```python
from build123d import *

# Parameters (mm, degrees)
SKETCH3_W = 0.254
SKETCH3_H = 0.508


with BuildPart() as part:
    # Sketch1 → Revolve1 (revolve)
    with BuildSketch(Plane.XY):
        Polygon((0, 0), (0, 1.5875), (1291.463, 1.5875), (1291.463, 4.03225), (1303.2994, 4.03225), (1303.2994, 0), align=None)
    revolve(axis=Axis((1303.2994, 0, 0), (-1, 0, 0)))

    # Sketch2 → Revolve2 (revolve)
    with BuildSketch(Plane.XY):
        Polygon((-9.652, 0), (-9.652, 1.20904), (-9.27354, 1.5875), (0, 1.5875), (0, 0), align=None)
    revolve(axis=Axis((0, 0, 0), (-1, 0, 0)))

    # Sketch3 → Cut-Revolve1 (revolve, cut)
    with BuildSketch(Plane.XY):
        with Locations((-0.127, 1.5875)):
            Rectangle(SKETCH3_W, SKETCH3_H)
    revolve(axis=Axis((0, 0, 0), (-1, 0, 0)), mode=Mode.SUBTRACT)


solid = part.part
```
Read the model definition and answer for the solid it produces. Units are mm, in the model's axes. Give positions to 0.01 mm unless a question says otherwise; leave off trailing zeros. Write each loop counter-clockwise with the first axis right and the second up, starting at its lowest first coordinate (ties: lowest second). Pieces come first, ordered by that corner, then holes. Notation, with made-up numbers: (26.5, 0) -> (62.5, 0) arc R21 cw to (62.5, 29) -> close; hole circle Ø1 at (55, 77.5). An arc over 180 degrees is marked (long way). Answer as a JSON object with one key per item and string values.
1) Flat-ended cylindrical pins translate along their axes: pin 1 Ø3 at (x, y) = (474.5, 2.5) entering from -Z; pin 2 Ø4 at (x, y) = (896, 2.5) entering from -Z; pin 3 Ø1.5 at (x, y) = (705.5, -1) entering from -Z; pin 4 Ø1 at (x, z) = (775, -3) entering from -Y. Find the tip coordinate at first contact, or state that the pin passes through.
Findings below:
{"pin 1": "stops at z = -1.23", "pin 2": "stops at z = -1.51", "pin 3": "stops at z = -1.57", "pin 4": "passes through"}
2) Straight lines are drawn through the part: probe 1 along X at (y, z) = (1, 1); probe 2 along X at (y, z) = (1.5, -1.5); probe 3 along Y at (x, z) = (773, 1.25). For each, find the intervals that lie inside material, in ascending order. Write a range as from..to.
Findings below:
{"probe 1": "x = -9.45..-0.25, 0..1303.3", "probe 2": "x = 1291.46..1303.3", "probe 3": "y = -0.98..0.98"}
3) Section A-A on x = 648 is taken. Write down the section's boundary in (y, z) (1 decimal), then the cut area to 3 significant figures.
Findings below:
{"outline": "circle Ø3.2 at (0, 0)", "area": "7.92 mm^2"}
